```python
from build123d import *

# Parameters (mm, degrees)
SKETCH1_R           = 2
BOSS_EXTRUDE1_DEPTH = 8
SKETCH2_W           = 24
SKETCH2_H           = 6
CUT_EXTRUDE1_DEPTH  = 2
SKETCH3_W           = 24
SKETCH3_H           = 6
CUT_EXTRUDE2_DEPTH  = 2
FILLET2_R           = 1
CHAMFER1_SIZE       = 1
CHAMFER2_SIZE       = 2
CHAMFER3_SIZE       = 2
CHAMFER5_SIZE       = 2
CHAMFER6_SIZE       = 2
CHAMFER7_SIZE       = 2
CHAMFER8_SIZE       = 2
CHAMFER9_SIZE       = 2
CHAMFER10_SIZE      = 2


with BuildPart() as part:
    # Sketch1 → Boss-Extrude1 (new body)
    with BuildSketch(Plane(origin=(0, 0, 0), x_dir=(1, 0, 0), z_dir=(0, 1, 0))):
        with BuildLine():
            Line((0, 7), (36, 7))
            ThreePointArc((36, 7), (43, 0), (36, -7))
            Line((36, -7), (0, -7))
            ThreePointArc((0, -7), (-0.043750855, -6.999863275), (-0.0875, -6.999453104))
            Line((-0.0875, -6.999453104), (-80.075, -5.999531232))
            ThreePointArc((-80.075, -5.999531232), (-86, 0), (-80.075, 5.999531232))
            Line((-80.075, 5.999531232), (-0.0875, 6.999453104))
            ThreePointArc((-0.0875, 6.999453104), (-0.043750855, 6.999863275), (0, 7))
        make_face()
        with Locations(Location((0, 0, 0), (0, 0, 270))):
            Circle(SKETCH1_R, mode=Mode.SUBTRACT)
        with Locations(Location((-80, 0, 0), (0, 0, 270))):
            Circle(SKETCH1_R, mode=Mode.SUBTRACT)
        with Locations(Location((36, 0, 0), (0, 0, 270))):
            Circle(SKETCH1_R, mode=Mode.SUBTRACT)
    extrude(amount=BOSS_EXTRUDE1_DEPTH)

    # Sketch2 → Cut-Extrude1 (cut)
    with BuildSketch(Plane(origin=(0, 8, 0), x_dir=(1, 0, 0), z_dir=(0, 1, 0))):
        Polygon((-74, 2.075162128), (-6, 2.925228542), (-6, -2.925228542), (-74, -2.075162128), align=None)
        with Locations((18, 0)):
            Rectangle(SKETCH2_W, SKETCH2_H)
    extrude(amount=-CUT_EXTRUDE1_DEPTH, mode=Mode.SUBTRACT)

    # Sketch3 → Cut-Extrude2 (cut)
    with BuildSketch(Plane.XZ):
        Polygon((-74, 2.075162128), (-6, 2.925228542), (-6, -2.925228542), (-74, -2.075162128), align=None)
        with Locations((18, 0)):
            Rectangle(SKETCH3_W, SKETCH3_H)
    extrude(amount=-CUT_EXTRUDE2_DEPTH, mode=Mode.SUBTRACT)

    # Fillet2
    fillet2_edges = [part.edges().sort_by_distance(p)[0] for p in [
        (-86, 8, 0),
        (-40.08125, 8, 6.499492168),
        (-0.043750855, 8, 6.999863275),
        (18, 8, 7),
        (43, 8, 0),
        (18, 8, -7),
        (-0.043750855, 8, -6.999863275),
        (-40.08125, 8, -6.499492168),
    ]]
    fillet(fillet2_edges, radius=FILLET2_R)

    # Chamfer1
    chamfer1_edges = [part.edges().sort_by_distance(p)[0] for p in [
        (-40.08125, 0, 6.499492168),
        (-86, 0, 0),
        (-40.08125, 0, -6.499492168),
        (-0.043750855, 0, -6.999863275),
        (18, 0, -7),
        (43, 0, 0),
        (18, 0, 7),
        (-0.043750855, 0, 6.999863275),
    ]]
    chamfer(chamfer1_edges, length=CHAMFER1_SIZE)

    # Chamfer2
    chamfer2_edges = [part.edges().sort_by_distance(p)[0] for p in [
        (18, 2, -3),
    ]]
    chamfer(chamfer2_edges, length=CHAMFER2_SIZE - 0.0001)  # a hair under: the kernel refuses the full size

    # Chamfer3
    chamfer3_edges = [part.edges().sort_by_distance(p)[0] for p in [
        (18, 2, 3),
    ]]
    chamfer(chamfer3_edges, length=CHAMFER3_SIZE - 0.0001)  # a hair under: the kernel refuses the full size

    # Chamfer5
    chamfer5_edges = [part.edges().sort_by_distance(p)[0] for p in [
        (-40, 2, -2.500195335),
    ]]
    chamfer(chamfer5_edges, length=CHAMFER5_SIZE - 0.0001)  # a hair under: the kernel refuses the full size

    # Chamfer6
    chamfer6_edges = [part.edges().sort_by_distance(p)[0] for p in [
        (-40, 2, 2.500195335),
    ]]
    chamfer(chamfer6_edges, length=CHAMFER6_SIZE - 0.0001)  # a hair under: the kernel refuses the full size

    # Chamfer7
    chamfer7_edges = [part.edges().sort_by_distance(p)[0] for p in [
        (-40, 6, -2.500195335),
    ]]
    chamfer(chamfer7_edges, length=CHAMFER7_SIZE - 0.0001)  # a hair under: the kernel refuses the full size

    # Chamfer8
    chamfer8_edges = [part.edges().sort_by_distance(p)[0] for p in [
        (18, 6, -3),
    ]]
    chamfer(chamfer8_edges, length=CHAMFER8_SIZE - 0.0001)  # a hair under: the kernel refuses the full size

    # Chamfer9
    chamfer9_edges = [part.edges().sort_by_distance(p)[0] for p in [
        (18, 6, 3),
    ]]
    chamfer(chamfer9_edges, length=CHAMFER9_SIZE - 0.0001)  # a hair under: the kernel refuses the full size

    # Chamfer10
    chamfer10_edges = [part.edges().sort_by_distance(p)[0] for p in [
        (-40, 6, 2.500195335),
    ]]
    chamfer(chamfer10_edges, length=CHAMFER10_SIZE - 0.0001)  # a hair under: the kernel refuses the full size


solid = part.part
```
For this review, take the finished solid that the model builds, in its own axes (mm). A direction names the side the tool comes from. Round coordinates to 2 decimals unless told otherwise and drop trailing zeros. Put each result on its own line as item: value.
Q1. Mouldability with a two-part tool opening along X and no side actions: class faces 4 (the face through (30, 1, 0)), 5 (the face through (42.2, 0.2, -0.1)), 6 (the face through (-85.2, 0.2, 0.1)), 7 (the face through (18, 1, 2)) as released by +X, released by -X, zero draft, split by the parting line, or undercut.
Solved:
face 4: undercut
face 5: released by +X
face 6: released by -X
face 7: undercut
Q2. Machinability: for faces 1 (the face through (-74, 1, 0)), 2 (the face through (18, 7, 2)), 3 (the face through (-39.52, 7.71, -6.21)), which of the approach directions +Z, -Z, +X, -X, +Y, -Y give a long, thin tool a straight path to every point of the face, cutting with its end or side? Answer none if there is none.
Solved:
face 1: -Y
face 2: +Y
face 3: -Z, -X, +Y
Q3. We need section A-A (y = 4.25). Count the separate pieces of the cut face and the enclosed holes in it, and give its area (3 significant figures).
Solved:
separate pieces: 1
enclosed holes: 3
area: 1,640 mm2
Q4. Insertion check: pin 1 Ø0.6 at (y, z) = (1.5, -0.5) entering from -X; pin 2 Ø3 at (x, y) = (-53, 4) entering from -Z; pin 3 Ø0.6 at (x, z) = (-24, -0.5) entering from +Y; pin 4 Ø3.5 at (x, z) = (36, 0) entering from +Y. Each pin has a flat end and moves straight along its axis. Give the tip position at first contact, or say it passes through.
Solved:
pin 1: stops at x = -86
pin 2: stops at z = -6.36
pin 3: stops at y = 6.1
pin 4: passes through
Q5. Wall thickness on probe 1 along X at (y, z) = (4.5, -1.75); probe 2 along Z at (x, y) = (16.5, 1.75); probe 3 along Z at (x, y) = (-25, 7): over which ranges is each line inside the solid? List them lowest first.
Solved:
probe 1: x = -85.74 to -80.97, -79.03 to -0.97, 0.97 to 35.03, 36.97 to 42.78
probe 2: z = -7 to -1.25, 1.25 to 7
probe 3: z = -6.69 to -1.69, 1.69 to 6.69
